```python
from build123d import *

# Parameters (mm, degrees)
SKETCH_1_W          = 37
SKETCH_1_H          = 40
EXTRUDE_1_DEPTH     = 2
SKETCH_2_W          = 2
SKETCH_2_H          = 20
EXTRUDE_2_DEPTH     = 4
SKETCH_3_R          = 1.05
CUT_EXTRUDE_1_DEPTH = 3
CUT_EXTRUDE_2_DEPTH = 10
FILLET_1_R          = 1.5


with BuildPart() as part:
    # 草图1 → 凸台-拉伸1 (new body)
    with BuildSketch(Plane.XY):
        Rectangle(SKETCH_1_W, SKETCH_1_H)
    extrude(amount=EXTRUDE_1_DEPTH)

    # 草图2 → 凸台-拉伸2 (add)
    with BuildSketch(Plane(origin=(18.5, 0, 0), x_dir=(0, 0, -1), z_dir=(1, 0, 0))):
        with Locations((-1, 1.2)):
            Rectangle(SKETCH_2_W, SKETCH_2_H)
    extrude_2 = extrude(amount=EXTRUDE_2_DEPTH)

    # 镜向1: 凸台-拉伸2 across plane
    add(extrude_2.mirror(Plane(origin=(0, 0, 0), x_dir=(0, 0, 1), z_dir=(1, 0, 0))))

    # 草图3 → 切除-拉伸1 (cut)
    with BuildSketch(Plane(origin=(0, 0, 0), x_dir=(-1, 0, 0), z_dir=(0, 0, -1))):
        with Locations((18.5, 12.25)):
            Circle(SKETCH_3_R)
        with Locations((18.5, -9.85)):
            Circle(SKETCH_3_R)
        with Locations((-18.5, -9.85)):
            Circle(SKETCH_3_R)
        with Locations((-18.5, 12.25)):
            Circle(SKETCH_3_R)
    extrude(amount=-CUT_EXTRUDE_1_DEPTH, mode=Mode.SUBTRACT)

    # 草图4 → 切除-拉伸2 (cut)
    with BuildSketch(Plane(origin=(0, 0, 0), x_dir=(-1, 0, 0), z_dir=(0, 0, -1))):
        Polygon((14.5, -1.713154672), (-11.394907157, -16), (14.5, -16), align=None)
        Polygon((-14.5, -1.5), (-14.5, -14.286845328), (8.676157157, -1.5), align=None)
        Polygon((-14.5, 14.286845328), (-14.5, 1.5), (8.676157157, 1.5), align=None)
        Polygon((-11.394907157, 16), (14.5, 1.713154672), (14.5, 16), align=None)
    extrude(amount=-CUT_EXTRUDE_2_DEPTH, mode=Mode.SUBTRACT)

    # 圆角1
    fillet_1_edges = [part.edges().sort_by_distance(p)[0] for p in [
        (11.394907157, 16, 1),
        (-14.5, 16, 1),
        (-14.5, 1.713154672, 1),
        (-14.5, -1.713154672, 1),
        (-14.5, -16, 1),
        (11.394907157, -16, 1),
        (18.5, -20, 1),
        (-18.5, -20, 1),
        (-18.5, 20, 1),
        (18.5, 20, 1),
        (14.5, -1.5, 1),
        (-8.676157157, -1.5, 1),
        (14.5, -14.286845328, 1),
        (14.5, 1.5, 1),
        (14.5, 14.286845328, 1),
        (-8.676157157, 1.5, 1),
    ]]
    fillet(fillet_1_edges, radius=FILLET_1_R)


solid = part.part
```
Source: CAD feature listing. Evaluate the final solid. Frame: model axes, mm. A direction names the side the tool comes from. Give positions to 0.01 mm unless a question says otherwise; leave off trailing zeros. Loops run counter-clockwise (first coordinate to the right, second up) from the corner with the lowest first, then second, coordinate; pieces in that order, holes last. Notation, with made-up numbers: M 27,40 L 40,40 A28 cw 40,75 Z; hole C 68,-2 d9. An arc over 180 degrees is marked long. Put each result on its own line as item: value.
Q1. Mould query, pull axis X, two halves, no side actions, for faces 4 (the flat face through (18.5, 16, 1)), 5 (the cylindrical face through (-14.07, -15.55, 1.01)), 6 (the flat face through (0, 0, 2)). Classes: released by +X, released by -X, zero draft, split by the parting line, or undercut.
Response values:
face 4: released by +X
face 5: undercut
face 6: zero draft
Q2. Section D-D (z = 0.8). Count the separate pieces of the cut face and the enclosed holes in it, and give its area (3 significant figures).
Response values:
separate pieces: 1
enclosed holes: 4
area: 996 mm²
Q3. Pin query (flat end, axial travel): P1, Ø1, axis at y = -14, z = 0.5, coming from the +X side; P2, Ø0.6, axis at y = 15, z = 0.5, coming from the -X side. Return the tip coordinate at first contact, or that it passes through.
Response values:
P1: stops at x = 18.5
P2: stops at x = -18.5
Q4. Line query: probe 1 along Y at (x, z) = (13, 1.5); probe 2 along X at (y, z) = (-6.5, 1.3); probe 3 along X at (y, z) = (6, 1.7). Output: solid intervals per line, ascending. Write a range as [from, to].
Response values:
probe 1: y = [-20, -13.25], [-1.5, 1.5], [13.25, 20]
probe 2: x = [-22.5, -14.5], [-5.82, 0.39], [14.5, 22.5]
probe 3: x = [-22.5, -14.5], [-6.73, -0.52], [14.5, 22.5]
Q5. Section C-C (x = 3). Return the cut outline in (y, z).
Response values:
outline: M -20,0 L -16,0 L -16,2 L -20,2 Z; M -11.37,0 L -7.94,0 L -7.94,2 L -11.37,2 Z; M -1.5,0 L 1.5,0 L 1.5,2 L -1.5,2 Z; M 7.94,0 L 11.37,0 L 11.37,2 L 7.94,2 Z; M 16,0 L 20,0 L 20,2 L 16,2 Z
Q6. Reachability of faces 1 (the flat face through (5, -1.5, 1)), 2 (the cylindrical face through (-17.45, -9.83, 0.99)), 3 (the flat face through (-18.5, 16, 1)) from +Z, -Z, +X, -X, +Y, -Y: full face, straight path, thin tool, end or side. Return the list, or none.
Response values:
face 1: +Z, -Z
face 2: +Z, -Z, -X
face 3: +Z, -Z, -X, +Y
Q7. Section A-A (x = 9.5). Return the cut outline in (y, z).
Response values:
outline: M -20,0 L -11.53,0 L -11.53,2 L -20,2 Z; M -1.5,0 L 1.5,0 L 1.5,2 L -1.5,2 Z; M 11.53,0 L 20,0 L 20,2 L 11.53,2 Z
Q8. Section B-B (y = -9.85). Return the cut outline in (x, z).
Response values:
outline: M -17.45,0 L -14.5,0 L -14.5,2 L -17.45,2 Z; M 0.25,0 L 6.46,0 L 6.46,2 L 0.25,2 Z; M 14.5,0 L 17.45,0 L 17.45,2 L 14.5,2 Z
